```python
from build123d import *

# Parameters (mm, degrees)
SKETCH1_R           = 1
BOSS_EXTRUDE1_DEPTH = 2.65


with BuildPart() as part:
    # Sketch1 → Boss-Extrude1 (new body)
    with BuildSketch(Plane(origin=(0, 0, 0), x_dir=(1, 0, 0), z_dir=(0, 1, 0))):
        with BuildLine():
            ThreePointArc((4.8, 6.9), (3.456497116, 6.343502884), (2.9, 5))
            Line((2.9, 5), (2.9, 1.4))
            ThreePointArc((2.9, 1.4), (2.753553391, 1.046446609), (2.4, 0.9))
            Line((2.4, 0.9), (2.214158983, 0.9))
            ThreePointArc((2.214158983, 0.9), (1.830463501, 0.720589734), (1.722123653, 0.311111111))
            ThreePointArc((1.722123653, 0.311111111), (0.604527333, -1.642268767), (-1.512826812, -0.879690308))
            ThreePointArc((-1.512826812, -0.879690308), (-1.628066031, -0.834192871), (-1.6991093, -0.935696311))
            Line((-1.6991093, -0.935696311), (-1.527088335, -3.928689929))
            ThreePointArc((-1.527088335, -3.928689929), (-1.371172257, -4.263555336), (-1.027912125, -4.4))
            Line((-1.027912125, -4.4), (1.5, -4.4))
            ThreePointArc((1.5, -4.4), (2.207106781, -4.692893219), (2.5, -5.4))
            Line((2.5, -5.4), (2.5, -5.9))
            ThreePointArc((2.5, -5.9), (2.792893219, -6.607106781), (3.5, -6.9))
            Line((3.5, -6.9), (5, -6.9))
            ThreePointArc((5, -6.9), (6.343502884, -6.343502884), (6.9, -5))
            Line((6.9, -5), (6.9, 5))
            ThreePointArc((6.9, 5), (6.343502884, 6.343502884), (5, 6.9))
            Line((5, 6.9), (4.8, 6.9))
        make_face()
        with Locations((5.5, 0)):
            Circle(SKETCH1_R, mode=Mode.SUBTRACT)
    extrude(amount=BOSS_EXTRUDE1_DEPTH)


solid = part.part
```
Input: part model. Units: mm. Frame: model coordinates. A direction names the side the tool comes from. Round coordinates to 2 decimals unless told otherwise and drop trailing zeros. Order: outer loops, then holes, each group sorted by start corner. A loop starts at its lowest first (then second) coordinate and runs counter-clockwise, first axis right, second up. Notation, with made-up numbers: (-31, 25) - (-20, 25) arc R17 ccw to (-20, 45) - close; hole circle Ø3 at (-4.5, 36). An arc over 180 degrees is marked (long way). Answer in a Markdown table with one row per item.
Item 1: Section query D-D (z = -3). Return the cut outline in (x, y), then the cut area to 3 significant figures.
Model answer:
| item | result |
|---|---|
| outline | (2.9, 0) - (6.9, 0) - (6.9, 2.65) - (2.9, 2.65) - close |
| area | 10.6 mm² |
Item 2: Section query C-C (y = 2.45). Return the cut outline in (x, z).
Model answer:
| item | result |
|---|---|
| outline | (-1.7, 0.94) arc R0.1 ccw to (-1.51, 0.88) arc R1.75 cw to (1.72, -0.31) arc R0.5 ccw to (2.21, -0.9) - (2.4, -0.9) arc R0.5 cw to (2.9, -1.4) - (2.9, -5) arc R1.9 ccw to (4.8, -6.9) - (5, -6.9) arc R1.9 ccw to (6.9, -5) - (6.9, 5) arc R1.9 ccw to (5, 6.9) - (3.5, 6.9) arc R1 ccw to (2.5, 5.9) - (2.5, 5.4) arc R1 cw to (1.5, 4.4) - (-1.03, 4.4) arc R0.5 ccw to (-1.53, 3.93) - close; hole circle Ø2 at (5.5, 0) |
Item 3: Line query: line 1 (X direction, y = 1.5, z = 0); line 2 (Z direction, x = 5.75, y = 2.55); line 3 (X direction, y = 2.2, z = 0.5). Output: solid intervals per line, ascending.
Model answer:
| item | result |
|---|---|
| line 1 | x = 1.75 to 4.5, 6.5 to 6.9 |
| line 2 | z = -6.75 to -0.97, 0.97 to 6.75 |
| line 3 | x = 1.68 to 4.63, 6.37 to 6.9 |
Item 4: Mould query, pull axis Z, two halves, no side actions, for faces 4 (the flat face through (-1.614, 1.306, 2.411)), 5 (the flat face through (4, 2.65, 0)), 6 (the cylindrical face through (4.7, 1.3, 0.6)), 7 (the cylindrical face through (6.358, 1.306, -6.329)). Classes: released by +Z, released by -Z, zero draft, split by the parting line, or undercut.
Model answer:
| item | result |
|---|---|
| face 4 | released by +Z |
| face 5 | zero draft |
| face 6 | undercut |
| face 7 | released by -Z |
Item 5: Pin query (flat end, axial travel): pin 1 (1.3 mm diameter, centred on x = 0.5, y = 1, fed in from +Z); pin 2 (0.8 mm diameter, centred on y = 2, z = -2.5, fed in from -X). Return the tip coordinate at first contact, or that it passes through.
Model answer:
| item | result |
|---|---|
| pin 1 | stops at z = 4.4 |
| pin 2 | stops at x = 2.9 |
Item 6: Reachability of faces 1 (the flat face through (0, 1, 4.4)), 2 (the flat face through (6.9, 1, 0)), 3 (the flat face through (2.9, 1, -3)) from +Z, -Z, +X, -X, +Y, -Y: full face, straight path, thin tool, end or side. Return the list, or none.
Model answer:
| item | result |
|---|---|
| face 1 | +Z, -X, +Y, -Y |
| face 2 | +Z, -Z, +X, +Y, -Y |
| face 3 | -Z, -X, +Y, -Y |
Item 7: Section query B-B (x = 5.5). Return the cut outline in (y, z), then the cut area to 3 significant figures.
Model answer:
| item | result |
|---|---|
| outline | (0, -6.83) - (2.65, -6.83) - (2.65, -1) - (0, -1) - close; (0, 1) - (2.65, 1) - (2.65, 6.83) - (0, 6.83) - close |
| area | 30.9 mm² |
Item 8: Section query A-A (z = 0). Return the cut outline in (x, y).
Model answer:
| item | result |
|---|---|
| outline | (1.75, 0) - (4.5, 0) - (4.5, 2.65) - (1.75, 2.65) - close; (6.5, 0) - (6.9, 0) - (6.9, 2.65) - (6.5, 2.65) - close |
